Check sheet for the modelled part. Datum: model origin and axes. Units: mm. Round coordinates to 2 decimals unless told otherwise and drop trailing zeros. Order: outer loops, then holes, each group sorted by start corner. A loop starts at its lowest first (then second) coordinate and runs counter-clockwise, first axis right, second up. Notation, with made-up numbers: (27, 6.25) -> (45, 6.25) arc R17 ccw to (45, 15.25) -> close; hole circle Ø10 at (-15, -9.75). An arc over 180 degrees is marked (long way). Answer in a Markdown table with one row per item.
from build123d import *
from build123d.topology import SkipClean

# Parameters (mm, degrees)
EXTRUDE_1_OUTLINE_R      = 45
EXTRUDE_1_OUTLINE_R_2    = 2.1
EXTRUDE_1_OUTLINE_R_3    = 1.6
EXTRUDE_1_OUTLINE_R_4    = 7.775
EXTRUDE_1_DEPTH          = 3
CUT_EXTRUDE_1_DEPTH      = 10
PATTERN_CIRCULAR_1_COUNT = 2
CUT_EXTRUDE_2_DEPTH      = 10
FILLET_1_R               = 2
CUT_EXTRUDE_3_REACH      = 65.71
SKETCH_4_R               = 1.4
CHAMFER_1_SIZE           = 1.1


# Read off the part's stored shape, not the designer's step: 凸台-拉伸1
with BuildPart() as part:
    # 凸台-拉伸1 outline → 凸台-拉伸1 (new body)
    with BuildSketch(Plane.XY):
        Circle(EXTRUDE_1_OUTLINE_R)
        with Locations((-29.69848481, -29.69848481)):
            Circle(EXTRUDE_1_OUTLINE_R_2, mode=Mode.SUBTRACT)
        with Locations((-17.320508076, -10)):
            Circle(EXTRUDE_1_OUTLINE_R_3, mode=Mode.SUBTRACT)
        with Locations((0, -42)):
            Circle(EXTRUDE_1_OUTLINE_R_2, mode=Mode.SUBTRACT)
        with Locations((29.69848481, -29.69848481)):
            Circle(EXTRUDE_1_OUTLINE_R_2, mode=Mode.SUBTRACT)
        with Locations((0, -20)):
            Circle(EXTRUDE_1_OUTLINE_R_3, mode=Mode.SUBTRACT)
        with Locations((17.320508076, -10)):
            Circle(EXTRUDE_1_OUTLINE_R_3, mode=Mode.SUBTRACT)
        with Locations((-42, 0)):
            Circle(EXTRUDE_1_OUTLINE_R_2, mode=Mode.SUBTRACT)
        with Locations((-17.320508076, 10)):
            Circle(EXTRUDE_1_OUTLINE_R_3, mode=Mode.SUBTRACT)
        with Locations((-29.69848481, 29.69848481)):
            Circle(EXTRUDE_1_OUTLINE_R_2, mode=Mode.SUBTRACT)
        Circle(EXTRUDE_1_OUTLINE_R_4, mode=Mode.SUBTRACT)
        with Locations((17.320508076, 10)):
            Circle(EXTRUDE_1_OUTLINE_R_3, mode=Mode.SUBTRACT)
        with Locations((0, 20)):
            Circle(EXTRUDE_1_OUTLINE_R_3, mode=Mode.SUBTRACT)
        with Locations((42, 0)):
            Circle(EXTRUDE_1_OUTLINE_R_2, mode=Mode.SUBTRACT)
        with Locations((0, 42)):
            Circle(EXTRUDE_1_OUTLINE_R_2, mode=Mode.SUBTRACT)
        with Locations((29.69848481, 29.69848481)):
            Circle(EXTRUDE_1_OUTLINE_R_2, mode=Mode.SUBTRACT)
    extrude(amount=EXTRUDE_1_DEPTH)

    # 草图2 → 切除-拉伸1 (cut)
    with BuildSketch(Plane.XY.offset(3)):
        with BuildLine():
            Line((4, 37.788887255), (4, 36.783148315))
            ThreePointArc((4, 36.783148315), (35.651970274, 9.896313233), (22.387428888, -29.4584967))
            Line((22.387428888, -29.4584967), (17.380966757, -24.452034569))
            ThreePointArc((17.380966757, -24.452034569), (16.963906124, -24.743198844), (16.541969004, -25.027250378))
            Line((16.541969004, -25.027250378), (22.290357636, -30.77563901))
            ThreePointArc((22.290357636, -30.77563901), (36.716063128, 9.794422308), (4, 37.788887255))
        make_face()
        with BuildLine():
            Line((-4, 37.788887255), (-4, 30.740852298))
            ThreePointArc((-4, 30.740852298), (26.614522572, 15.895508431), (25.168841559, -18.097773747))
            Line((25.168841559, -18.097773747), (24.452034569, -17.380966757))
            ThreePointArc((24.452034569, -17.380966757), (25.41530796, 15.93932625), (-5, 29.580398915))
            Line((-5, 29.580398915), (-5, 37.669616404))
            ThreePointArc((-5, 37.669616404), (-4.500395136, 37.732564763), (-4, 37.788887255))
        make_face()
    cut_extrude_1 = extrude(amount=-CUT_EXTRUDE_1_DEPTH, mode=Mode.SUBTRACT)

    # 阵列(圆周)1: 切除-拉伸1 ×2 about axis
    pattern_circular_1_axis = Axis((0, 0, 0), (0, 0, 1))
    for i in range(1, PATTERN_CIRCULAR_1_COUNT):
        add(cut_extrude_1.rotate(pattern_circular_1_axis, i * 360 / PATTERN_CIRCULAR_1_COUNT), mode=Mode.SUBTRACT)

    # 草图3 → 切除-拉伸2 (cut)
    with SkipClean():  # the faces are left unmerged after this step: merging them gives an invalid solid
        with BuildSketch(Plane.XY.offset(3)):
            with BuildLine():
                Line((-5, 37.669616404), (-5, 29.580398915))
                ThreePointArc((-5, 29.580398915), (-11.00894625, 27.907043958), (-16.541969004, 25.027250378))
                Line((-16.541969004, 25.027250378), (-22.290357636, 30.77563901))
                ThreePointArc((-22.290357636, 30.77563901), (-14.073828052, 35.297696298), (-5, 37.669616404))
            make_face()
            with BuildLine():
                Line((16.541969004, -25.027250378), (22.290357636, -30.77563901))
                ThreePointArc((22.290357636, -30.77563901), (14.073828052, -35.297696298), (5, -37.669616404))
                Line((5, -37.669616404), (5, -29.580398915))
                ThreePointArc((5, -29.580398915), (11.00894625, -27.907043958), (16.541969004, -25.027250378))
            make_face()
        extrude(amount=-CUT_EXTRUDE_2_DEPTH, mode=Mode.SUBTRACT)

    # 圆角1
    fillet_1_edges = [part.edges().sort_by_distance(p)[0] for p in [
        (4, -37.788887255, 1.5),
        (4, -30.740852298, 1.5),
        (-17.380966757, 24.452034569, 1.5),
        (-22.387428888, 29.4584967, 1.5),
        (-4, 37.788887255, 1.5),
        (-4, 30.740852298, 1.5),
        (17.380966757, -24.452034569, 1.5),
        (22.387428888, -29.4584967, 1.5),
    ]]
    fillet(fillet_1_edges, radius=FILLET_1_R)

    # 草图4 → 切除-拉伸3 (cut, up to next)
    with BuildSketch(Plane(origin=(0, 0, 0), x_dir=(-1, 0, 0), z_dir=(0, 0, -1)), mode=Mode.PRIVATE) as cut_extrude_3_sk1:
        with Locations((0, 12.5)):
            Circle(SKETCH_4_R)
    cut_extrude_3_tool1 = extrude(cut_extrude_3_sk1.sketch, amount=-CUT_EXTRUDE_3_REACH, mode=Mode.PRIVATE) & part.part
    # 草图4 → 切除-拉伸3 (cut, up to next)
    with BuildSketch(Plane(origin=(0, 0, 0), x_dir=(-1, 0, 0), z_dir=(0, 0, -1)), mode=Mode.PRIVATE) as cut_extrude_3_sk2:
        with Locations((10.825317547, 6.25)):
            Circle(SKETCH_4_R)
    cut_extrude_3_tool2 = extrude(cut_extrude_3_sk2.sketch, amount=-CUT_EXTRUDE_3_REACH, mode=Mode.PRIVATE) & part.part
    # 草图4 → 切除-拉伸3 (cut, up to next)
    with BuildSketch(Plane(origin=(0, 0, 0), x_dir=(-1, 0, 0), z_dir=(0, 0, -1)), mode=Mode.PRIVATE) as cut_extrude_3_sk3:
        with Locations((10.825317547, -6.25)):
            Circle(SKETCH_4_R)
    cut_extrude_3_tool3 = extrude(cut_extrude_3_sk3.sketch, amount=-CUT_EXTRUDE_3_REACH, mode=Mode.PRIVATE) & part.part
    # 草图4 → 切除-拉伸3 (cut, up to next)
    with BuildSketch(Plane(origin=(0, 0, 0), x_dir=(-1, 0, 0), z_dir=(0, 0, -1)), mode=Mode.PRIVATE) as cut_extrude_3_sk4:
        with Locations((0, -12.5)):
            Circle(SKETCH_4_R)
    cut_extrude_3_tool4 = extrude(cut_extrude_3_sk4.sketch, amount=-CUT_EXTRUDE_3_REACH, mode=Mode.PRIVATE) & part.part
    # 草图4 → 切除-拉伸3 (cut, up to next)
    with BuildSketch(Plane(origin=(0, 0, 0), x_dir=(-1, 0, 0), z_dir=(0, 0, -1)), mode=Mode.PRIVATE) as cut_extrude_3_sk5:
        with Locations((-10.825317547, -6.25)):
            Circle(SKETCH_4_R)
    cut_extrude_3_tool5 = extrude(cut_extrude_3_sk5.sketch, amount=-CUT_EXTRUDE_3_REACH, mode=Mode.PRIVATE) & part.part
    # 草图4 → 切除-拉伸3 (cut, up to next)
    with BuildSketch(Plane(origin=(0, 0, 0), x_dir=(-1, 0, 0), z_dir=(0, 0, -1)), mode=Mode.PRIVATE) as cut_extrude_3_sk6:
        with Locations((-10.825317547, 6.25)):
            Circle(SKETCH_4_R)
    cut_extrude_3_tool6 = extrude(cut_extrude_3_sk6.sketch, amount=-CUT_EXTRUDE_3_REACH, mode=Mode.PRIVATE) & part.part
    add(cut_extrude_3_tool1.solids().sort_by_distance((0, 12.5, 0))[0], mode=Mode.SUBTRACT)
    add(cut_extrude_3_tool2.solids().sort_by_distance((-10.825318, 6.25, 0))[0], mode=Mode.SUBTRACT)
    add(cut_extrude_3_tool3.solids().sort_by_distance((-10.825318, -6.25, 0))[0], mode=Mode.SUBTRACT)
    add(cut_extrude_3_tool4.solids().sort_by_distance((0, -12.5, 0))[0], mode=Mode.SUBTRACT)
    add(cut_extrude_3_tool5.solids().sort_by_distance((10.825318, -6.25, 0))[0], mode=Mode.SUBTRACT)
    add(cut_extrude_3_tool6.solids().sort_by_distance((10.825318, 6.25, 0))[0], mode=Mode.SUBTRACT)

    # 倒角1
    chamfer_1_edges = [part.edges().sort_by_distance(p)[0] for p in [
        (1.4, 12.5, 0),
        (12.225317547, 6.25, 0),
        (12.225317547, -6.25, 0),
        (1.4, -12.5, 0),
        (-9.425317547, -6.25, 0),
        (-9.425317547, 6.25, 0),
    ]]
    chamfer(chamfer_1_edges, length=CHAMFER_1_SIZE)


solid = part.part
Item 1: Cross-section at B-B (x = 0). State how many separate pieces and enclosed holes the cut face has, and give its area (3 significant figures).
Result sheet:
| item | result |
|---|---|
| separate pieces | 10 |
| enclosed holes | 0 |
| area | 154 mm^2 |
Item 2: Mould release check, pull along X, two halves, no side actions. Record for faces 1 (the flat face through (-1, -9, 3)), 2 (the cylindrical face through (20.765, -39.923, 1.479)), 3 (the flat face through (-4, 34, 2)): pulls with the +X half, pulls with the -X half, needs draft (parallel to the pull), parting line crosses it, or undercut.
Result sheet:
| item | result |
|---|---|
| face 1 | needs draft |
| face 2 | parting line crosses it |
| face 3 | undercut |
Item 3: Scan lines: line 1 (Y direction, x = 33, z = 1.35); line 2 (Y direction, x = -10, z = 2.5); line 3 (X direction, y = -14.5, z = 2.65). Record each from-to range of solid material in increasing order. Write a range as [from, to].
Result sheet:
| item | result |
|---|---|
| line 1 | y = [-30.59, -18.84], [-16.73, 16.73], [18.84, 30.59] |
| line 2 | y = [-43.87, -36.66], [-35.62, -29.34], [-28.28, -7.38], [-5.12, 5.12], [7.38, 28.28], [36.66, 43.87] |
| line 3 | x = [-42.6, -35.12], [-34.04, -27.4], [-26.26, 26.26], [27.4, 34.04], [35.12, 42.6] |
Item 4: Depth check by flat-ended pin: P1, Ø4, axis at x = 29.7, y = 29.7, coming from the -Z side; P2, Ø0.8, axis at y = 34, z = 2, coming from the -X side; P3, Ø1.5, axis at y = -20.5, z = 2, coming from the +X side; P4, Ø1.5, axis at y = -36, z = 0.5, coming from the +X side. Enter the tip coordinate at first touch or a pass-through.
Result sheet:
| item | result |
|---|---|
| P1 | passes through |
| P2 | stops at x = -29.93 |
| P3 | stops at x = 40.43 |
| P4 | stops at x = 27.97 |
Item 5: Cross-section at A-A (y = 20). Record the boundary of the cut face in (x, z), and give its area (3 significant figures).
Result sheet:
| item | result |
|---|---|
| outline | (-40.31, 0) -> (-32.31, 0) -> (-32.31, 3) -> (-40.31, 3) -> close; (-31.13, 0) -> (-1.6, 0) -> (-1.6, 3) -> (-31.13, 3) -> close; (1.6, 0) -> (22.36, 0) -> (22.36, 3) -> (1.6, 3) -> close; (23.69, 0) -> (31.13, 0) -> (31.13, 3) -> (23.69, 3) -> close; (32.31, 0) -> (40.31, 0) -> (40.31, 3) -> (32.31, 3) -> close |
| area | 221 mm^2 |
